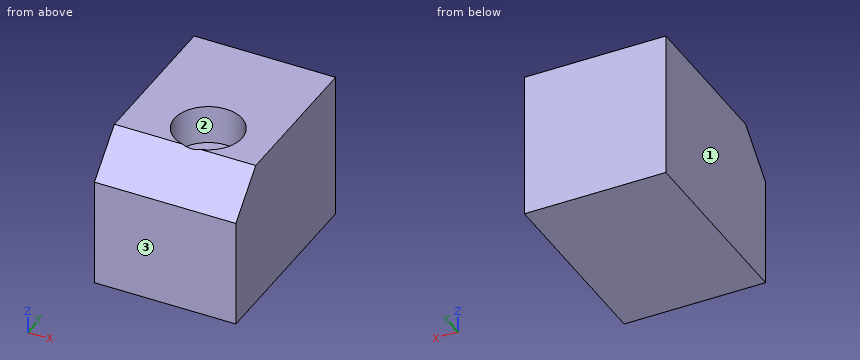
```python
from build123d import *

# Parameters (mm, degrees)
F0_W        = 92.6014147699
F0_H        = 96.5672135353
F1_DEPTH    = 127
F2_R        = 22.1483335528
F3_DEPTH    = 25.4
F4_T1_DEPTH = 223.2429105586


# Not quite as in the source:
# - a fillet or chamfer that OpenCascade refuses, or shapes differently, is made with other operations: its cross-section is extruded or revolved along the edge and cut away or added


with BuildPart() as f1:
    # F0 (on Front) → F1 (new body)
    with BuildSketch(Plane.XZ):
        with Locations((0.2974327654, -0.594869256)):
            Rectangle(F0_W, F0_H)
    extrude(amount=F1_DEPTH)

    # F2 (on face) → F3 (cut)
    with BuildSketch(Plane.XY.offset(47.6887375116)):
        with Locations((4.5238654129, -80.271743238)):
            Circle(F2_R)
    extrude(amount=-F3_DEPTH, mode=Mode.SUBTRACT)

    # F4: chamfer of 25.4 on 1 edges, made by hand

    # F4_s2 → F4_t1 (cut)
    with BuildSketch(Plane.YZ.offset(-111.3240225139)):
        Polygon((-101.6, 47.6887375116), (-127, 22.2887375116), (-127, 47.6887375116), align=None)
    extrude(amount=F4_T1_DEPTH, mode=Mode.SUBTRACT)


solid = f1.part
```
Here's how the part is built. I have some questions about the finished solid (model axes, mm). Face numbers are marked on the shaded views. Coordinates: 2 decimals unless noted, no trailing zeros. Loops run counter-clockwise (first coordinate to the right, second up) from the corner with the lowest first, then second, coordinate; pieces in that order, holes last. Notation, with made-up numbers: (71, 2) - (116, 2) arc R7 cw to (116, 6) - close; hole circle Ø1 at (22, 45.5). An arc over 180 degrees is marked (long way). Return JSON: item names as keys, results as strings. Group by question number.
Item 1: If we section it at C-C on x = 18: Write out the boundary of the cut face in (y, z), and give its area (3 significant figures).
Item 2: I need wall thicknesses on line 1 (Z direction, x = -7.5, y = -74); line 2 (X direction, y = -88, z = 36); line 3 (Y direction, x = -36, z = 24). Which ranges of each line are inside material? Lowest first, please. Write a range as from..to.
Item 3: If we section it at A-A on x = -34: Write out the boundary of the cut face in (y, z).
Item 4: If we section it at D-D on y = -68.5: Write out the boundary of the cut face in (x, z).
Item 5: We'd pull the mould along X, two halves only. Please class the marked faces 1, 2 and 3: +X half, -X half, draft (parallel to the pull), parting line (faces both ways), or undercut.
Item 6: Will these pins go through, and if not, where does the flat tip stop? P1, Ø22, axis at x = -0.5, y = -83, coming from the +Z side; P2, Ø3, axis at x = 10, z = 22.5, coming from the -Y side.
Item 7: If we section it at B-B on y = -97.5: Write out the boundary of the cut face in (x, z), and give its area (3 significant figures).
Calculated:
{
 "1": {"outline": "(-127, -48.88) - (0, -48.88) - (0, 47.69) - (-62.69, 47.69) - (-62.69, 22.29) - (-97.85, 22.29) - (-97.85, 47.69) - (-101.6, 47.69) - (-127, 22.29) - close", "area": "11,000 mm^2"},
 "2": {"line 1": "z = -48.88..22.29", "line 2": "x = -46..-16.23, 25.28..46.6", "line 3": "y = -125.29..0"},
 "3": {"outline": "(-127, -48.88) - (0, -48.88) - (0, 47.69) - (-101.6, 47.69) - (-127, 22.29) - close"},
 "4": {"outline": "(-46, -48.88) - (46.6, -48.88) - (46.6, 47.69) - (23.28, 47.69) - (23.28, 22.29) - (-14.24, 22.29) - (-14.24, 47.69) - (-46, 47.69) - close"},
 "5": {"face 1": "-X half", "face 2": "undercut", "face 3": "draft"},
 "6": {"P1": "stops at z = 22.29", "P2": "stops at y = -127"},
 "7": {"outline": "(-46, -48.88) - (46.6, -48.88) - (46.6, 47.69) - (18.44, 47.69) - (18.44, 22.29) - (-9.4, 22.29) - (-9.4, 47.69) - (-46, 47.69) - close", "area": "8,240 mm^2"}
}
